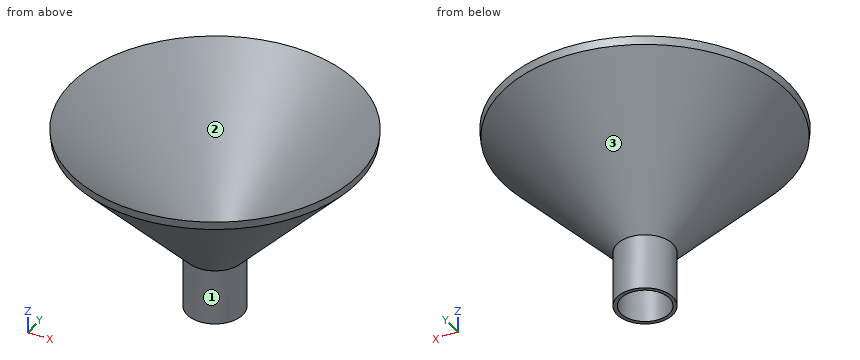
```python
from build123d import *

# Parameters (mm, degrees)
F2_R     = 11.019259
F3_DEPTH = 50.8
F4_DEPTH = 25.4


with BuildPart() as f1:
    # F0 (on Front) → F1 (revolve)
    with BuildSketch(Plane.XZ):
        Polygon((0, -25.4), (0, 0), (52.254206, 55.461139), (52.654178, 59.21939), (-1.341835, 1.909547), (-12.7, 1.909547), (-12.7, -25.4), align=None)
    revolve(axis=Axis((-12.7, 0, -11.745227), (0, 0, 1)))

    # F2 (on Top) → F3 (cut)
    with BuildSketch(Plane.XY):
        with Locations((-12.766276, 0)):
            Circle(F2_R)
    extrude(amount=-F3_DEPTH, mode=Mode.SUBTRACT)

    # F2 (on Top) → F4 (cut)
    with BuildSketch(Plane.XY):
        with Locations((-12.766276, 0)):
            Circle(F2_R)
    extrude(amount=F4_DEPTH, mode=Mode.SUBTRACT)


solid = f1.part
```
Read the model definition and answer for the solid it produces. Units are mm, in the model's axes. Face numbers are marked on the shaded views. Give positions to 0.01 mm unless a question says otherwise; leave off trailing zeros. Order: outer loops, then holes, each group sorted by start corner. A loop starts at its lowest first (then second) coordinate and runs counter-clockwise, first axis right, second up. Notation, with made-up numbers: (-27, 60.5) -> (22, 60.5) arc R27 ccw to (22, 96.5) -> close; hole circle Ø4 at (-28.5, 22). An arc over 180 degrees is marked (long way). One line per item, written item: value. Start each with the question number.
(1) Straight lines are drawn through the part: L1, parallel to Y at x = -53.5, z = 48; L2, parallel to Y at x = -5, z = 16; L3, parallel to X at y = -6, z = 49.5. For each, find the intervals that lie inside material, in ascending order.
(2) Flat-ended cylindrical pins translate along their axes: P1, Ø1.5, axis at x = -10.5, z = 6, coming from the -Y side; P2, Ø3, axis at x = 8, y = -47, coming from the +Z side; P3, Ø12, axis at x = 17, y = 33, coming from the -Z side. Find the tip coordinate at first contact, or state that the pin passes through.
(3) The part is cut by section D-D (z = 41.5). Determine the outline of the cut face in (x, y), and give its area (3 significant figures).
(4) The part is cut by section B-B (x = -12.7). Determine the outline of the cut face in (y, z).
(5) The part is cut by section C-C (z = -7). Determine the outline of the cut face in (x, y).
(6) For a pull along Z with two mould halves and no side action, classify the marked faces 1, 2 and 3 as released by +Z, released by -Z, zero draft, split by the parting line, or undercut.
(7) The part is cut by section A-A (y = 0). Determine the outline of the cut face in (x, z), and give its area (3 significant figures).
Taken from the geometry:
1. L1: -41.12 to -36.56, 36.56 to 41.12
1. L2: -26.69 to -23.4, 23.4 to 26.69
1. L3: -71.73 to -68.58, 43.18 to 46.33
2. P1: y = -18.94
2. P2: z = 45.95
2. P3: z = 27.27
3. outline: circle Ø103.6 at (-12.7, 0); hole circle Ø97.32 at (-12.7, 0)
3. area: 991 mm^2
4. outline: (-65.35, 59.22) -> (-64.95, 55.46) -> (-12.7, 0) -> (-12.7, -25.4) -> (-11.02, -25.4) -> (-11.02, 1.91) -> (-11.36, 1.91) -> close; (11.02, -25.4) -> (12.7, -25.4) -> (12.7, 0) -> (64.95, 55.46) -> (65.35, 59.22) -> (11.36, 1.91) -> (11.02, 1.91) -> close
5. outline: circle Ø25.4 at (-12.7, 0); hole circle Ø22.04 at (-12.77, 0)
6. face 1: zero draft
6. face 2: released by +Z
6. face 3: released by -Z
7. outline: (-78.05, 59.22) -> (-77.65, 55.46) -> (-25.4, 0) -> (-25.4, -25.4) -> (-23.79, -25.4) -> (-23.79, 1.91) -> (-24.06, 1.91) -> close; (-1.75, -25.4) -> (0, -25.4) -> (0, 0) -> (52.25, 55.46) -> (52.65, 59.22) -> (-1.34, 1.91) -> (-1.75, 1.91) -> close
7. area: 443 mm^2
